Can you work these out from the model? Positions are in its coordinate system, mm. Face numbers are marked on the shaded views. A direction names the side the tool comes from. Round coordinates to 2 decimals unless told otherwise and drop trailing zeros. Write each loop counter-clockwise with the first axis right and the second up, starting at its lowest first coordinate (ties: lowest second). Pieces come first, ordered by that corner, then holes. Notation, with made-up numbers: M 56,42.5 L 94,42.5 A33 cw 94,77.5 Z; hole C 64.5,-35.75 d4. An arc over 180 degrees is marked long. Answer in a Markdown table with one row per item. Add a question column.
(1) If we mould it in two halves opening along Z, with no side actions, what happens to the marked faces 1, 2 and 3? For each: released by +Z, released by -Z, zero draft, split by the parting line, or undercut.
(2) For the marked faces 4 and 5, which set-ups out of +Z, -Z, +X, -X, +Y, -Y let a thin tool reach every point of the face, with its end or its side?
(3) I'm going to push flat-ended pins straight in: pin 1 (20.5 mm diameter, centred on x = -11, y = 37.5, fed in from -Z); pin 2 (4 mm diameter, centred on y = 43, z = -17, fed in from -X); pin 3 (5 mm diameter, centred on x = 17, z = -16, fed in from +Y); pin 4 (2.5 mm diameter, centred on x = -13.5, z = 9, fed in from +Y). Where does each tip first touch, or does it pass through?
(4) Suppose I cut it at B-B, the plane z = -1.5. Write out the boundary of the cut face in (x, y), then the cut area to 3 significant figures.
(5) If I drill on probe 1 along X at (y, z) = (0.6, -14); probe 2 along X at (y, z) = (46.5, -15); probe 3 along X at (y, z) = (1, 11), over which ranges is the centre line in solid material (lowest first)?
(6) Suppose I cut it at A-A, the plane y = 27.5. Write out the boundary of the cut face in (x, z), then the cut area to 3 significant figures.
(7) Suppose I cut it at C-C, the plane y = 43. Write out the boundary of the cut face in (x, z).
(8) Suppose I cut it at D-D, the plane x = 9. Write out the boundary of the cut face in (y, z).
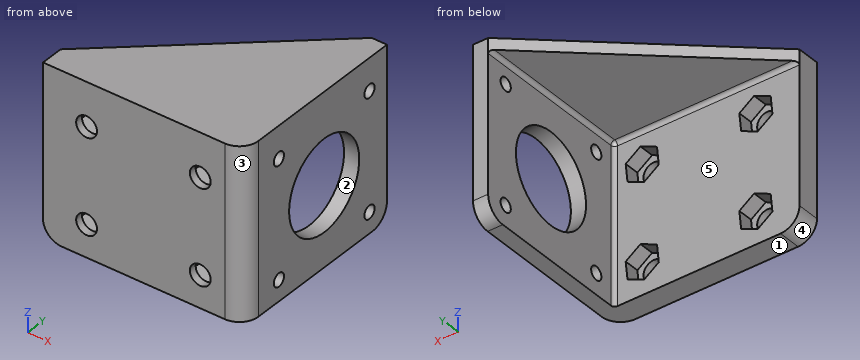
from build123d import *

# Parameters (mm, degrees)
ESBO_O1_W                = 53
ESBO_O1_H                = 45
RESSALTO_EXTRUS_O1_DEPTH = 6
ESBO_O2_W                = 4
ESBO_O2_H                = 45
RESSALTO_EXTRUS_O2_DEPTH = 43
RESSALTO_EXTRUS_O3_DEPTH = 3
ESBO_O4_R                = 12
ESBO_O4_R_2              = 1.75
CORTE_EXTRUS_O1_DEPTH    = 73.857738093
ESBO_O5_R                = 2.75
CORTE_EXTRUS_O2_DEPTH    = 56.294665204
FILETE1_R                = 5
FILETE2_R                = 1
CORTE_EXTRUS_O4_DEPTH    = 4
FILETE3_R                = 5


with BuildPart() as part:
    # Esboço1 → Ressalto-extrusão1 (new body)
    with BuildSketch(Plane(origin=(0, 0, 0), x_dir=(1, 0, 0), z_dir=(0, 1, 0))):
        Rectangle(ESBO_O1_W, ESBO_O1_H)
    extrude(amount=RESSALTO_EXTRUS_O1_DEPTH)

    # Esboço2 → Ressalto-extrusão2 (add)
    with BuildSketch(Plane(origin=(0, 6, 0), x_dir=(1, 0, 0), z_dir=(0, 1, 0))):
        with Locations((24.5, 0)):
            Rectangle(ESBO_O2_W, ESBO_O2_H)
    extrude(amount=RESSALTO_EXTRUS_O2_DEPTH)

    # Esboço3 → Ressalto-extrusão3 (add)
    with BuildSketch(Plane.XY.offset(22.5)):
        Polygon((-26.5, 6), (22.5, 49), (22.5, 6), align=None)
    extrude(amount=-RESSALTO_EXTRUS_O3_DEPTH)

    # Esboço4 → Corte-extrusão1 (cut, through all)
    with BuildSketch(Plane.ZY.offset(-22.5)):
        with Locations((-1.5, 27.5)):
            Circle(ESBO_O4_R)
        with Locations((-17, 43)):
            Circle(ESBO_O4_R_2)
        with Locations((14, 43)):
            Circle(ESBO_O4_R_2)
        with Locations((14, 12)):
            Circle(ESBO_O4_R_2)
        with Locations((-17, 12)):
            Circle(ESBO_O4_R_2)
    extrude(amount=-CORTE_EXTRUS_O1_DEPTH, mode=Mode.SUBTRACT)

    # Esboço5 → Corte-extrusão2 (cut, through all)
    with BuildSketch(Plane(origin=(0, 6, 0), x_dir=(1, 0, 0), z_dir=(0, 1, 0))):
        with Locations(Location((-15, 14, 0), (0, 0, 270))):
            Circle(ESBO_O5_R)
        with Locations(Location((-15, -11, 0), (0, 0, 270))):
            Circle(ESBO_O5_R)
        with Locations(Location((15, -11, 0), (0, 0, 90))):
            Circle(ESBO_O5_R)
        with Locations(Location((15, 14, 0), (0, 0, 90))):
            Circle(ESBO_O5_R)
    extrude(amount=-CORTE_EXTRUS_O2_DEPTH, mode=Mode.SUBTRACT)

    # Filete1
    filete1_edges = [part.edges().sort_by_distance(p)[0] for p in [
        (24.5, 49, -22.5),
        (-26.5, 3, -22.5),
    ]]
    fillet(filete1_edges, radius=FILETE1_R)

    # Filete2
    filete2_edges = [part.edges().sort_by_distance(p)[0] for p in [
        (22.5, 6, -1.5),
        (-2, 6, 19.5),
        (22.5, 27.5, 19.5),
    ]]
    fillet(filete2_edges, radius=FILETE2_R)

    # Esboço7 → Corte-extrusão4 (cut)
    with BuildSketch(Plane(origin=(0, 6, 0), x_dir=(1, 0, 0), z_dir=(0, 1, 0))):
        Polygon((15.473054225, 9.231399258), (19.366256495, 12.025376605), (18.89320227, 16.793977347), (14.526945775, 18.768600742), (10.633743505, 15.974623395), (11.10679773, 11.206022653), align=None)
        Polygon((-14.526945775, 9.231399258), (-10.633743505, 12.025376605), (-11.10679773, 16.793977347), (-15.473054225, 18.768600742), (-19.366256495, 15.974623395), (-18.89320227, 11.206022653), align=None)
        Polygon((15.473054225, -15.768600742), (19.366256495, -12.974623395), (18.89320227, -8.206022653), (14.526945775, -6.231399258), (10.633743505, -9.025376605), (11.10679773, -13.793977347), align=None)
        Polygon((-14.526945775, -15.768600742), (-10.633743505, -12.974623395), (-11.10679773, -8.206022653), (-15.473054225, -6.231399258), (-19.366256495, -9.025376605), (-18.89320227, -13.793977347), align=None)
    extrude(amount=-CORTE_EXTRUS_O4_DEPTH, mode=Mode.SUBTRACT)

    # Filete3
    filete3_edges = [part.edges().sort_by_distance(p)[0] for p in [
        (26.5, 0, 0),
    ]]
    fillet(filete3_edges, radius=FILETE3_R)


solid = part.part
Calculated:
| question | item | result |
|---|---|---|
| 1 | face 1 | released by -Z |
| 1 | face 2 | undercut |
| 1 | face 3 | zero draft |
| 2 | face 4 | -Z, -X, +Y, -Y |
| 2 | face 5 | -Z, -X, +Y |
| 3 | pin 1 | through |
| 3 | pin 2 | x = 22.5 |
| 3 | pin 3 | y = 6 |
| 3 | pin 4 | y = 2 |
| 4 | outline | M -26.5,0 L 21.5,0 A5 ccw 26.5,5 L 26.5,15.5 L 22.5,15.5 L 22.5,7 A1 cw 21.5,6 L -26.5,6 Z; M 22.5,39.5 L 26.5,39.5 L 26.5,49 L 22.5,49 Z |
| 4 | area | 389 mm² |
| 5 | probe 1 | -26.5 to -17.75, -12.25 to 12.25, 17.75 to 23.87 |
| 5 | probe 2 | 22.5 to 26.5 |
| 5 | probe 3 | -26.5 to -17.75, -12.25 to 12.25, 17.75 to 24.5 |
| 6 | outline | M -2,19.5 L 21.5,19.5 A1 cw 22.5,18.5 L 22.5,10.5 L 26.5,10.5 L 26.5,22.5 L -2,22.5 Z; M 22.5,-22.5 L 26.5,-22.5 L 26.5,-13.5 L 22.5,-13.5 Z |
| 6 | area | 158 mm² |
| 7 | outline | M 15.66,19.5 L 21.5,19.5 A1 cw 22.5,18.5 L 22.5,15.75 L 26.5,15.75 L 26.5,22.5 L 15.66,22.5 Z; M 22.5,-22.5 L 26.5,-22.5 L 26.5,-18.75 L 22.5,-18.75 Z; M 22.5,-15.25 L 26.5,-15.25 L 26.5,12.25 L 22.5,12.25 Z |
| 8 | outline | M 0,-22.5 L 6,-22.5 L 6,18.5 A1 cw 7,19.5 L 37.15,19.5 L 37.15,22.5 L 0,22.5 Z |
